from build123d import *

# Parameters (mm, degrees)
F0_W        = 40
F0_H        = 40
F1_DEPTH    = 40
F2_W        = 29.62
F2_H        = 29.62
F3_DEPTH    = 29.62
F4_T1_DEPTH = 65.7168298797
F4_T3_DEPTH = 65.7168298797


# Not quite as in the source:
# - a fillet or chamfer that OpenCascade refuses, or shapes differently, is made with other operations: its cross-section is extruded or revolved along the edge and cut away or added


with BuildPart() as f1:
    # F0 (on Top) → F1 (new body)
    with BuildSketch(Plane.XY):
        with Locations((20, 20)):
            Rectangle(F0_W, F0_H)
    extrude(amount=F1_DEPTH)

    # F2 (on face) → F3 (cut)
    with BuildSketch(Plane.XY.offset(40)):
        with Locations((19.9230909348, 19.5811167631)):
            Rectangle(F2_W, F2_H)
    extrude(amount=-F3_DEPTH, mode=Mode.SUBTRACT)

    # F4: chamfer of 5 on 4 edges, made by hand

    # F4_s2 → F4_t1 (cut)
    with BuildSketch(Plane.YZ.offset(-12.8584149398)):
        Polygon((0, 35), (5, 40), (0, 40), align=None)
        Polygon((40, 35), (35, 40), (40, 40), align=None)
    extrude(amount=F4_T1_DEPTH, mode=Mode.SUBTRACT)

    # F4_s4 → F4_t3 (cut)
    with BuildSketch(Plane.XZ.offset(-52.8584149398)):
        Polygon((35, 40), (40, 35), (40, 40), align=None)
        Polygon((0, 35), (5, 40), (0, 40), align=None)
    extrude(amount=F4_T3_DEPTH, mode=Mode.SUBTRACT)


solid = f1.part
Read the model definition and answer for the solid it produces. Units are mm, in the model's axes. A direction names the side the tool comes from. Give positions to 0.01 mm unless a question says otherwise; leave off trailing zeros. Write each loop counter-clockwise with the first axis right and the second up, starting at its lowest first coordinate (ties: lowest second). Pieces come first, ordered by that corner, then holes. Notation, with made-up numbers: M -19,80 L 33,80 A17 cw 33,90 Z; hole C -38,70.5 d4. An arc over 180 degrees is marked long. One line per item, written item: value. Start each with the question number.
(1) Find the intervals of material crossed by line 1 (Y direction, x = 19, z = 11); line 2 (X direction, y = 21.5, z = 35); line 3 (Z direction, x = 23, y = 12), in increasing order.
(2) Find section B-B (y = 7). Determine the outline of the cut face in (x, z), plus the area to 3 significant figures.
(3) Determine the mould class of faces 3 (the flat face through (34.733, 19, 25)), 4 (the flat face through (20, 38, 37)), 5 (the flat face through (37, 20, 38)) for opening direction X: pulls with the +X half, pulls with the -X half, needs draft (parallel to the pull), parting line crosses it, or undercut.
(4) Find section C-C (x = 13.5). Determine the outline of the cut face in (y, z).
(5) Find section D-D (z = 11). Determine the outline of the cut face in (x, y), plus the area to 3 significant figures.
(6) Find section A-A (z = 36.5). Determine the outline of the cut face in (x, y), plus the area to 3 significant figures.
(7) A flat-ended cylindrical pin translates along its axis: pin 1 Ø15 at (x, y) = (23, 24) entering from +Z. Find the tip coordinate at first contact, or state that the pin passes through.
(8) A tool of negligible diameter and unlimited length cuts with its end or side. For faces 1 (the flat face through (5.113, 19, 25)), 2 (the flat face through (0, 20, 17)), from which of +Z, -Z, +X, -X, +Y, -Y can it reach the whole face along a straight path? Write none if from no direction.
Results below:
1. line 1: y = 0 to 4.77, 34.39 to 40
1. line 2: x = 0 to 5.11, 34.73 to 40
1. line 3: z = 0 to 10.38
2. outline: M 0,0 L 40,0 L 40,35 L 35,40 L 34.73,40 L 34.73,10.38 L 5.11,10.38 L 5.11,40 L 5,40 L 0,35 Z
2. area: 698 mm^2
3. face 3: undercut
3. face 4: needs draft
3. face 5: pulls with the +X half
4. outline: M 0,0 L 40,0 L 40,35 L 35,40 L 34.39,40 L 34.39,10.38 L 4.77,10.38 L 4.77,39.77 L 0,35 Z
5. outline: M 0,0 L 40,0 L 40,40 L 0,40 Z; hole M 5.11,4.77 L 34.73,4.77 L 34.73,34.39 L 5.11,34.39 Z
5. area: 723 mm^2
6. outline: M 1.5,1.5 L 38.5,1.5 L 38.5,38.5 L 1.5,38.5 Z; hole M 5.11,4.77 L 34.73,4.77 L 34.73,34.39 L 5.11,34.39 Z
6. area: 492 mm^2
7. pin 1: stops at z = 10.38
8. face 1: +Z
8. face 2: +Z, -Z, -X, +Y, -Y
